Here's how the part is built. I have some questions about the finished solid (model axes, mm). A direction names the side the tool comes from. Give positions to 0.01 mm unless a question says otherwise; leave off trailing zeros. Loops run counter-clockwise (first coordinate to the right, second up) from the corner with the lowest first, then second, coordinate; pieces in that order, holes last. Notation, with made-up numbers: (-21, 67) - (18, 67) arc R12 cw to (18, 80) - close; hole circle Ø9 at (45, 70). An arc over 180 degrees is marked (long way). Use one line per item in the form item = value.
from build123d import *

# Parameters (mm, degrees)
PAD007_DEPTH      = 2.5
PAD008_DEPTH      = 5
PAD009_DEPTH      = 3.2
CYLINDER001_R     = 1.75
CYLINDER001_DEPTH = 8.5
FILLET004_R       = 1
CYLINDER002_R     = 3
CYLINDER002_DEPTH = 4
PAD011_DEPTH      = 8.5
FILLET005_R       = 1
PAD012_DEPTH      = 4
PAD013_DEPTH      = 7
PAD014_DEPTH      = 4
POCKET003_DEPTH   = 3.5


with BuildPart() as part:
    # Sketch009 (on DatumPlane) → Pad007 (new body)
    with BuildSketch(Plane.XY.offset(-82.8)):
        with BuildLine():
            Line((-76.8, 46.8), (76.8, 46.8))
            Line((76.8, 46.8), (76.8, -40))
            ThreePointArc((70, -46.8), (74.808326, -44.808326), (76.8, -40))
            Line((70, -46.8), (-75, -46.8))
            ThreePointArc((-76.8, -45), (-76.272792, -46.272792), (-75, -46.8))
            Line((-76.8, -45), (-76.8, 46.8))
        make_face()
    extrude(amount=PAD007_DEPTH)

    # Sketch010 (on DatumPlane) → Pad008 (join)
    with BuildSketch(Plane(origin=(57.5, 19.5, -80.3), x_dir=(1, 0, 0), z_dir=(0, 0, 1))):
        Polygon((-11.8, 26.5), (-13.8, 26.5), (-13.8, -28.8), (13.8, -28.8), (13.8, 26.5), (11.8, 26.5), (11.8, -26.8), (-11.8, -26.8), align=None)
    extrude(amount=PAD008_DEPTH)

    # Sketch011 (on DatumPlane) → Pad009 (join)
    with BuildSketch(Plane.XY.offset(-80.3)):
        Polygon((45.7, 46), (47.5, 46), (47.5, -6.3), (67.5, -6.3), (67.5, 46), (69.3, 46), (69.3, -7.3), (45.7, -7.3), align=None)
    extrude(amount=PAD009_DEPTH)

    # Cylinder001 → Cylinder001 (join)
    with BuildSketch(Plane(origin=(24, -19, -80.3), x_dir=(1, 0, 0), z_dir=(0, 0, 1))):
        Circle(CYLINDER001_R)
    extrude(amount=CYLINDER001_DEPTH)

    # Fillet004
    fillet004_edges = [part.edges().sort_by_distance(p)[0] for p in [
        (22.25, -19, -71.8),
    ]]
    fillet(fillet004_edges, radius=FILLET004_R)

    # Cylinder002 → Cylinder002 (join)
    with BuildSketch(Plane(origin=(24, -19, -80.3), x_dir=(1, 0, 0), z_dir=(0, 0, 1))):
        Circle(CYLINDER002_R)
    extrude(amount=CYLINDER002_DEPTH)

    # Sketch016 (on Face1 of Cylinder002) → Pad011 (join)
    with BuildSketch(Plane(origin=(24, -19, -80.3), x_dir=(1, 0, 0), z_dir=(0, 0, 1))):
        with BuildLine():
            ThreePointArc((-50, 1.75), (-51.75, 0), (-50, -1.75))
            Line((-50, -1.75), (-47, -1.75))
            ThreePointArc((-47, -1.75), (-45.25, 0), (-47, 1.75))
            Line((-47, 1.75), (-50, 1.75))
        make_face()
    extrude(amount=PAD011_DEPTH)

    # Fillet005
    fillet005_edges = [part.edges().sort_by_distance(p)[0] for p in [
        (-24.5, -20.75, -71.8),
        (-27.75, -19, -71.8),
        (-24.5, -17.25, -71.8),
        (-21.25, -19, -71.8),
    ]]
    fillet(fillet005_edges, radius=FILLET005_R)

    # Sketch017 (on Face4 of Fillet005) → Pad012 (join)
    with BuildSketch(Plane.XY.offset(-80.3)):
        with BuildLine():
            ThreePointArc((-26, -16), (-29, -19), (-26, -22))
            Line((-26, -22), (-23, -22))
            ThreePointArc((-23, -22), (-20, -19), (-23, -16))
            Line((-23, -16), (-26, -16))
        make_face()
    extrude(amount=PAD012_DEPTH)

    # Sketch018 (on Face1 of Pad012) → Pad013 (join)
    with BuildSketch(Plane.XY.offset(-80.3)):
        Polygon((31.8, -32.3), (31.8, -42.3), (16.8, -42.3), (16.8, -44.8), (34.3, -44.8), (34.3, -32.3), align=None)
        Polygon((-31.8, -5.7), (-31.8, 4.3), (-16.8, 4.3), (-16.8, 6.8), (-34.3, 6.8), (-34.3, -5.7), align=None)
        Polygon((16.8, 4.3), (16.8, 6.8), (34.3, 6.8), (34.3, -5.7), (31.8, -5.7), (31.8, 4.3), align=None)
        Polygon((-31.8, -32.3), (-34.3, -32.3), (-34.3, -44.8), (-16.8, -44.8), (-16.8, -42.3), (-31.8, -42.3), align=None)
    extrude(amount=PAD013_DEPTH)

    # Sketch019 (on Face1 of Pad013) → Pad014 (join)
    with BuildSketch(Plane.XY.offset(-80.3)):
        Polygon((18.8, 1.8), (18.8, 4.3), (31.8, 4.3), (31.8, -0.088908), (29.3, -0.088908), (29.3, 1.8), align=None)
        Polygon((-31.8, -3.7), (-29.3, -3.7), (-29.3, 1.8), (-18.8, 1.8), (-18.8, 4.3), (-31.8, 4.3), align=None)
        Polygon((-31.8, -42.3), (-31.8, -34.3), (-29.3, -34.3), (-29.3, -39.8), (-18.8, -39.8), (-18.8, -42.3), align=None)
        Polygon((31.8, -34.3), (29.3, -34.3), (29.3, -39.8), (18.8, -39.8), (18.8, -42.3), (31.8, -42.3), align=None)
    extrude(amount=PAD014_DEPTH)

    # Sketch020 (on Face1 of Pad014) → Pocket003 (cut)
    with BuildSketch(Plane.XY.offset(-80.3)):
        with BuildLine():
            ThreePointArc((2, -15.5), (0, -13.5), (-2, -15.5))
            Line((-2, -15.5), (-2, -22.5))
            ThreePointArc((-2, -22.5), (0, -24.5), (2, -22.5))
            Line((2, -22.5), (2, -15.5))
        make_face()
        with BuildLine():
            ThreePointArc((-2, -7.705551), (0, -9.705551), (2, -7.705551))
            Line((2, -7.705551), (2, -0.705551))
            ThreePointArc((2, -0.705551), (0, 1.294449), (-2, -0.705551))
            Line((-2, -0.705551), (-2, -7.705551))
        make_face()
        with BuildLine():
            ThreePointArc((-2, -37.294449), (0, -39.294449), (2, -37.294449))
            Line((2, -37.294449), (2, -30.294449))
            ThreePointArc((2, -30.294449), (0, -28.294449), (-2, -30.294449))
            Line((-2, -30.294449), (-2, -37.294449))
        make_face()
        with BuildLine():
            ThreePointArc((-13.590624, -15.5), (-15.590624, -13.5), (-17.590624, -15.5))
            Line((-17.590624, -15.5), (-17.590624, -22.5))
            ThreePointArc((-17.590624, -22.5), (-15.590624, -24.5), (-13.590624, -22.5))
            Line((-13.590624, -22.5), (-13.590624, -15.5))
        make_face()
        with BuildLine():
            ThreePointArc((-17.590624, -7.705551), (-15.590624, -9.705551), (-13.590624, -7.705551))
            Line((-13.590624, -7.705551), (-13.590624, -0.705551))
            ThreePointArc((-13.590624, -0.705551), (-15.590624, 1.294449), (-17.590624, -0.705551))
            Line((-17.590624, -0.705551), (-17.590624, -7.705551))
        make_face()
        with BuildLine():
            ThreePointArc((-17.590624, -37.294449), (-15.590624, -39.294449), (-13.590624, -37.294449))
            Line((-13.590624, -37.294449), (-13.590624, -30.294449))
            ThreePointArc((-13.590624, -30.294449), (-15.590624, -28.294449), (-17.590624, -30.294449))
            Line((-17.590624, -30.294449), (-17.590624, -37.294449))
        make_face()
        with BuildLine():
            ThreePointArc((17.590624, -15.5), (15.590624, -13.5), (13.590624, -15.5))
            Line((13.590624, -15.5), (13.590624, -22.5))
            ThreePointArc((13.590624, -22.5), (15.590624, -24.5), (17.590624, -22.5))
            Line((17.590624, -22.5), (17.590624, -15.5))
        make_face()
        with BuildLine():
            ThreePointArc((13.590624, -7.705551), (15.590624, -9.705551), (17.590624, -7.705551))
            Line((17.590624, -7.705551), (17.590624, -0.705551))
            ThreePointArc((17.590624, -0.705551), (15.590624, 1.294449), (13.590624, -0.705551))
            Line((13.590624, -0.705551), (13.590624, -7.705551))
        make_face()
        with BuildLine():
            ThreePointArc((13.590624, -37.294449), (15.590624, -39.294449), (17.590624, -37.294449))
            Line((17.590624, -37.294449), (17.590624, -30.294449))
            ThreePointArc((17.590624, -30.294449), (15.590624, -28.294449), (13.590624, -30.294449))
            Line((13.590624, -30.294449), (13.590624, -37.294449))
        make_face()
        with BuildLine():
            ThreePointArc((-5.795312, -7.363847), (-7.795312, -5.363847), (-9.795312, -7.363847))
            Line((-9.795312, -7.363847), (-9.795312, -14.363847))
            ThreePointArc((-9.795312, -14.363847), (-7.795312, -16.363847), (-5.795312, -14.363847))
            Line((-5.795312, -14.363847), (-5.795312, -7.363847))
        make_face()
        with BuildLine():
            ThreePointArc((-9.795312, -30.636153), (-7.795312, -32.636153), (-5.795312, -30.636153))
            Line((-5.795312, -30.636153), (-5.795312, -23.636153))
            ThreePointArc((-5.795312, -23.636153), (-7.795312, -21.636153), (-9.795312, -23.636153))
            Line((-9.795312, -23.636153), (-9.795312, -30.636153))
        make_face()
        with BuildLine():
            ThreePointArc((9.795312, -7.363847), (7.795312, -5.363847), (5.795312, -7.363847))
            Line((5.795312, -7.363847), (5.795312, -14.363847))
            ThreePointArc((5.795312, -14.363847), (7.795312, -16.363847), (9.795312, -14.363847))
            Line((9.795312, -14.363847), (9.795312, -7.363847))
        make_face()
        with BuildLine():
            ThreePointArc((5.795312, -30.636153), (7.795312, -32.636153), (9.795312, -30.636153))
            Line((9.795312, -30.636153), (9.795312, -23.636153))
            ThreePointArc((9.795312, -23.636153), (7.795312, -21.636153), (5.795312, -23.636153))
            Line((5.795312, -23.636153), (5.795312, -30.636153))
        make_face()
    extrude(amount=-POCKET003_DEPTH, mode=Mode.SUBTRACT)


solid = part.part
(1) If we section it at B-B (y = -12): List the corners of the cut face in (x, z) for me, plus the area to 3 significant figures.
Geometry says:
outline = (-76.8, -82.8) - (-9.8, -82.8) - (-9.8, -80.3) - (-76.8, -80.3) - close; (-5.8, -82.8) - (5.8, -82.8) - (5.8, -80.3) - (-5.8, -80.3) - close; (9.8, -82.8) - (76.8, -82.8) - (76.8, -80.3) - (9.8, -80.3) - close
area = 364 mm²
(2) For faces 5 (the flat face through (-34.3, -38, -77)), 6 (the flat face through (-31.8, -36, -75)), 7 (the flat face through (-25, -20.75, -75)), which set-ups out of +Z, -Z, +X, -X, +Y, -Y let a thin tool reach every point of the face, with its end or its side?
Geometry says:
face_5 = +Z, -X, +Y, -Y
face_6 = +Z
face_7 = +Z, +X, -X
(3) For P1, Ø1.6, axis at y = 21, z = -79, coming from the +X side; P2, Ø3.5, axis at y = 23, z = -78.5, coming from the -X side; P3, Ø4.5, axis at x = -22.5, z = -79, coming from the -Y side; P4, Ø2.5, axis at x = -33, z = -78.5, coming from the -Y side, each with a flat end and sliding along its axis, tell me the tip position at first contact or that it passes through.
Geometry says:
P1 = 71.3
P2 = 43.7
P3 = -46.8
P4 = -44.8
(4) If we section it at A-A (x = 0): List the corners of the cut face in (y, z) for me.
Geometry says:
outline = (-46.8, -82.8) - (-39.29, -82.8) - (-39.29, -80.3) - (-46.8, -80.3) - close; (-28.29, -82.8) - (-24.5, -82.8) - (-24.5, -80.3) - (-28.29, -80.3) - close; (-13.5, -82.8) - (-9.71, -82.8) - (-9.71, -80.3) - (-13.5, -80.3) - close; (1.29, -82.8) - (46.8, -82.8) - (46.8, -80.3) - (1.29, -80.3) - close
(5) If I drill on probe 1 along X at (y, z) = (4, -80); probe 2 along X at (y, z) = (-38, -77.25); probe 3 along X at (y, z) = (-25, -81), over which ranges is the centre line in solid material (lowest first)?
Geometry says:
probe_1 = -34.3 to -18.8, 18.8 to 34.3, 43.7 to 47.5, 67.5 to 71.3
probe_2 = -34.3 to -29.3, 29.3 to 34.3
probe_3 = -76.8 to -9.8, -5.8 to 5.8, 9.8 to 76.8
(6) Thinking about a two-plate mould opening in X: for faces 1 (the flat face through (69, 46, -78)), 2 (the flat face through (71.3, 18, -78)), 3 (the flat face through (-24, -42.3, -75)), 4 (the flat face through (-24, 1.8, -78)), which applies, pulls with the +X half, pulls with the -X half, needs draft (parallel to the pull), parting line crosses it, or undercut?
Geometry says:
face_1 = needs draft
face_2 = pulls with the +X half
face_3 = undercut
face_4 = undercut
